Autodesk Inventor part; units mm, degrees
ref_plane "YZ Plane" through (0, 0, 0) normal (1, 0, 0) x (0, 1, 0)
ref_plane "XZ Plane" through (0, 0, 0) normal (0, 1, 0) x (-1, 0, 0)
ref_plane "XY Plane" through (0, 0, 0) normal (0, 0, 1) x (1, 0, 0)
sketch "Arduino Uno" plane through (0, 0, 0) normal (0, 0, 1) x (1, 0, 0)
  line L0 (0, 0) -> (68.6, 0)
  line L1 (68.6, 0) -> (68.6, 53.3)
  line L2 (68.6, 53.3) -> (0, 53.3)
  line L3 (0, 53.3) -> (0, 0)
  circle A0 centre (14, 2.5) radius 1.6
  circle A1 centre (66.1, 7.6) radius 1.6
  circle A2 centre (66.1, 35.5) radius 1.6
  circle A3 centre (15.3, 50.7) radius 1.6
  dimension "d6" = 68.6
  dimension "d7" = 53.3
  dimension "d34" = 3.2
  dimension "d35" = 2.5
  dimension "d36" = 14
  dimension "d37" = 3.2
  dimension "d38" = 66.1
  dimension "d39" = 7.6
  dimension "d40" = 3.2
  dimension "d41" = 35.5
  dimension "d42" = 66.1
  dimension "d43" = 3.2
  dimension "d44" = 15.3
  dimension "d45" = 50.7
sketch "Sketch2" plane through (0, 0, 0) normal (0, 0, 1) x (1, 0, 0)
  line L0 (0, 0) -> (8, 0)
  line L1 (-2.2793, -6.7051) -> (-2.2793, 63.2949)
  line L2 (-2.2793, 63.2949) -> (77.7207, 63.2949)
  line L3 (77.7207, 63.2949) -> (77.7207, -6.7051)
  line L4 (77.7207, -6.7051) -> (-2.2793, -6.7051)
  dimension "d27" = 8
  dimension "d28" = 70
  dimension "d29" = 80
extrude "Back Plate" add sketch "Sketch2" against normal blind 5
extrude "Uno Mounting Holes" cut sketch "Arduino Uno" against normal through all contours A0 | A1 | A2 | A3
properties part number "UNO-Mounting-Holes"
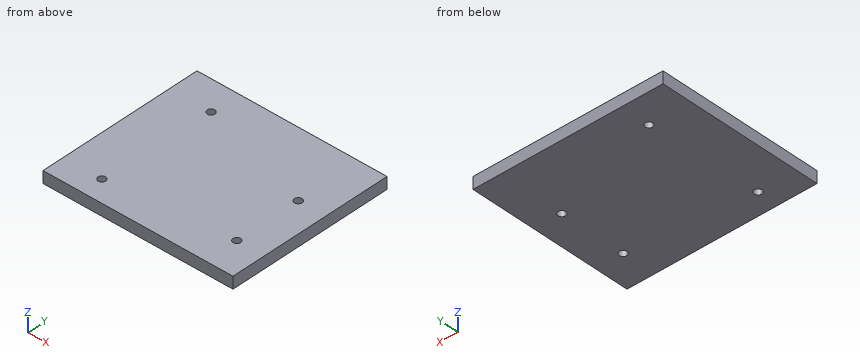
Here's how the part is built. I have some questions about the finished solid (model axes, mm). Round coordinates to 2 decimals unless told otherwise and drop trailing zeros. Order: outer loops, then holes, each group sorted by start corner. A loop starts at its lowest first (then second) coordinate and runs counter-clockwise, first axis right, second up. Notation, with made-up numbers: M 65,54 L 77,54 A27 ccw 77,85 Z; hole C -28.5,28.25 d5. An arc over 180 degrees is marked long. Answer in a Markdown table with one row per item.
Item 1: If I drill on L1, parallel to Y at x = 14, z = -1.35, over which ranges is the centre line in solid material (lowest first)? Write a range as from..to.
A:
| item | result |
|---|---|
| L1 | y = -6.71..0.9, 4.1..49.77, 51.63..63.29 |
Item 2: Imagine slicing it at B-B, the plane y = 35.5. Write out the boundary of the cut face in (x, z), and give its area (3 significant figures).
A:
| item | result |
|---|---|
| outline | M -2.28,-5 L 64.5,-5 L 64.5,0 L -2.28,0 Z; M 67.7,-5 L 77.72,-5 L 77.72,0 L 67.7,0 Z |
| area | 384 mm2 |
Item 3: Imagine slicing it at A-A, the plane x = 66.1. Write out the boundary of the cut face in (y, z).
A:
| item | result |
|---|---|
| outline | M -6.71,-5 L 6,-5 L 6,0 L -6.71,0 Z; M 9.2,-5 L 33.9,-5 L 33.9,0 L 9.2,0 Z; M 37.1,-5 L 63.29,-5 L 63.29,0 L 37.1,0 Z |
Item 4: I'm going to push a flat-ended pin straight in: pin 1 (2.5 mm diameter, centred on x = 15.3, y = 50.7, fed in from +Z). Where does the tip first touch, or does it pass through?
A:
| item | result |
|---|---|
| pin 1 | passes through |
